Can you work these out from the drawing? Everything is in mm from the part's minimum corner. Give positions to 0.01 mm unless a question says otherwise; leave off trailing zeros. Order: outer loops, then holes, each group sorted by start corner. A loop starts at its lowest first (then second) coordinate and runs counter-clockwise, first axis right, second up. Notation, with made-up numbers: (-5.5, 80) - (18.5, 80) arc R15 cw to (18.5, 100) - close; hole circle Ø8 at (23, -12.5). An arc over 180 degrees is marked (long way). Answer as a JSON object with one key per item and string values.
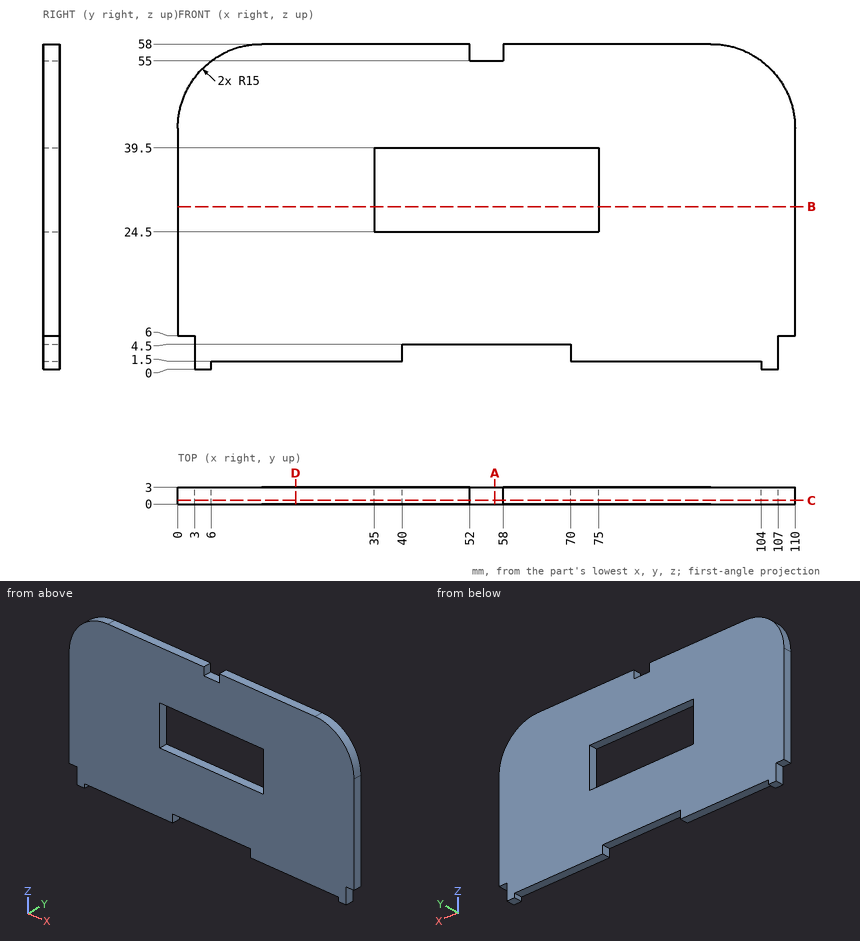
Q1. I need wall thicknesses on L1, parallel to Z at x = 71.5, y = 2.5; L2, parallel to X at y = 1.85, z = 27; L3, parallel to Z at x = 58.5, y = 2.7. Which ranges of each line are inside material? Lowest first, please.
Recorded:
{"L1": "z = 1.5 to 24.5, 39.5 to 58", "L2": "x = 0 to 35, 75 to 110", "L3": "z = 4.5 to 24.5, 39.5 to 58"}
Q2. If we section it at C-C, the plane y = 0.7: Please give me the cut outline in (x, z).
Recorded:
{"outline": "(0, 6) - (3, 6) - (3, 0) - (6, 0) - (6, 1.5) - (40, 1.5) - (40, 4.5) - (70, 4.5) - (70, 1.5) - (104, 1.5) - (104, 0) - (107, 0) - (107, 6) - (110, 6) - (110, 43) arc R15 ccw to (95, 58) - (58, 58) - (58, 55) - (52, 55) - (52, 58) - (15, 58) arc R15 ccw to (0, 43) - close; hole (35, 24.5) - (75, 24.5) - (75, 39.5) - (35, 39.5) - close"}
Q3. If we section it at D-D, the plane x = 21: Please give me the cut outline in (y, z).
Recorded:
{"outline": "(0, 1.5) - (3, 1.5) - (3, 58) - (0, 58) - close"}
Q4. I'm going to push flat-ended pins straight in: pin 1 Ø0.9 at (x, y) = (109, 1) entering from -Z; pin 2 Ø0.9 at (x, y) = (84.5, 1.5) entering from -Z; pin 3 Ø1.5 at (x, y) = (55, 2) entering from +Z. Where does each tip first touch, or does it pass through?
Recorded:
{"pin 1": "stops at z = 6", "pin 2": "stops at z = 1.5", "pin 3": "stops at z = 55"}
Q5. If we section it at B-B, the plane z = 29: Please give me the cut outline in (x, y).
Recorded:
{"outline": "(0, 0) - (35, 0) - (35, 3) - (0, 3) - close; (75, 0) - (110, 0) - (110, 3) - (75, 3) - close"}
Q6. If we section it at A-A, the plane x = 56.5: Please give me the cut outline in (y, z).
Recorded:
{"outline": "(0, 4.5) - (3, 4.5) - (3, 24.5) - (0, 24.5) - close; (0, 39.5) - (3, 39.5) - (3, 55) - (0, 55) - close"}
